Geometry check sheet. Reference: the model listing, model coordinates, mm. A direction names the side the tool comes from. Give positions to 0.01 mm unless a question says otherwise; leave off trailing zeros. Order: outer loops, then holes, each group sorted by start corner. A loop starts at its lowest first (then second) coordinate and runs counter-clockwise, first axis right, second up. Notation, with made-up numbers: M 67,55 L 101,55 A14 ccw 101,69 Z; hole C -19.5,43 d2. An arc over 180 degrees is marked long. Answer as CSV lines item,"result". Start each with the question number.
Q1. Set-up check for faces 1 (the flat face through (2, 4, -1)), 2 (the flat face through (1.8, 3.4, 1.9)), 3 (the flat face through (0, 2, 1)): record each of +Z, -Z, +X, -X, +Y, -Y from which the full face is reachable in a straight line by a thin tool's end or side.
Q2. Go/stop test with flat-tipped pins: pin 1 (1.8 mm diameter, centred on x = 4, z = 2.5, fed in from +Y); pin 2 (0.5 mm diameter, centred on y = 3.5, z = 2.5, fed in from +X); pin 3 (2 mm diameter, centred on x = 4, z = 1.5, fed in from +Y). Record where each tip stops, or that it passes through.
Q3. Thickness scan on line 1 (Y direction, x = 3.7, z = 1); line 2 (Y direction, x = 0.9, z = 1); line 3 (Z direction, x = 4.2, y = 0.25). Record the ranges inside material, lowest first.
Q4. Section check A-A, the plane y = 2.7. Record the boundary of the cut face in (x, z), then the cut area to 3 significant figures.
```python
from build123d import *

# Parameters (mm, degrees)
BOSS_EXTRUDE1_DEPTH = 3.2
BOSS_EXTRUDE2_DEPTH = 1.8
BOSS_EXTRUDE3_DEPTH = 3.2


with BuildPart() as part:
    # Sketch1 → Boss-Extrude1 (new body)
    with BuildSketch(Plane(origin=(0, 0, 0), x_dir=(0, 0, -1), z_dir=(1, 0, 0))):
        with BuildLine():
            Line((2.000388773, 4), (-0.998443773, 4))
            Line((-0.998443773, 4), (-0.998443773, 1.094743417))
            add(Edge.make_bspline(
                [(2.000388773, 0), (0.565989501, 1.139941433), (-0.998443773, 1.094743417)],
                knots=[0, 0, 0, 0.519824709, 0.519824709, 0.519824709], degree=2))
            Line((2.000388773, 0), (2.000388773, 4))
        make_face()
    extrude(amount=BOSS_EXTRUDE1_DEPTH)

    # Sketch2 → Boss-Extrude2 (add)
    with BuildSketch(Plane.ZY):
        with BuildLine():
            add(Edge.make_bspline(
                [(0.998443773, 1.094743417), (2.014440988, 1.074460094), (3.030499337, 0.688991657), (3.999611226, 0)],
                knots=[0.49982829, 0.49982829, 0.49982829, 0.49982829, 1, 1, 1, 1], degree=3))
            Line((3.999611227, 0), (3.999611226, 0.998709843))
            ThreePointArc((3.999611226, 0.998709843), (3.120597073, 3.120899083), (0.998443773, 4))
            Line((0.998443773, 4), (0.998443773, 1.094743417))
        make_face()
    extrude(amount=-BOSS_EXTRUDE2_DEPTH)

    # Sketch3 → Boss-Extrude3 (add)
    with BuildSketch(Plane(origin=(1.8, 0, 0), x_dir=(0, 0, -1), z_dir=(1, 0, 0))):
        with BuildLine():
            add(Edge.make_bspline(
                [(-3.999611227, 0), (-3.02996408, 0.689665176), (-2.014175759, 1.074793835), (-0.998443773, 1.094743417)],
                knots=[0, 0, 0, 0, 0.50017171, 0.50017171, 0.50017171, 0.50017171], degree=3))
            Line((-0.998443773, 1.094743417), (-0.998443773, 3))
            Line((-0.998443773, 3), (-3.234965952, 3))
            ThreePointArc((-3.234965952, 3), (-3.801940417, 2.069905984), (-3.999611226, 0.998709843))
            Line((-3.999611227, 0.998709843), (-3.999611227, 0))
        make_face()
        with BuildLine():
            add(Edge.make_bspline(
                [(-0.998443773, 1.094743417), (0.016590806, 1.114679302), (1.031569126, 0.769937407), (2.000388773, 0)],
                knots=[0.50017171, 0.50017171, 0.50017171, 0.50017171, 1, 1, 1, 1], degree=3))
            Line((2.000388773, 0), (2.000388773, 5.000856569))
            add(Edge.make_bspline(
                [(2.000388773, 5.000856569), (1.39753578, 2.931475432), (-0.998443773, 3)],
                knots=[0, 0, 0, 1, 1, 1], degree=2))
            Line((-0.998443773, 3), (-0.998443773, 1.094743417))
        make_face()
    extrude(amount=BOSS_EXTRUDE3_DEPTH)


solid = part.part
```
Answer block:
1,face 1,"+Z, -X, +Y"
1,face 2,"+Z, +X, +Y"
1,face 3,"+Z, -Z, -X, +Y, -Y"
2,pin 1,"stops at y = 3"
2,pin 2,"stops at x = 1.8"
2,pin 3,"stops at y = 4"
3,line 1,"y = 1.09 to 3"
3,line 2,"y = 1.09 to 4"
3,line 3,"z = -2 to -1.66, 3.62 to 4"
4,outline,"M 0,-2 L 5,-2 L 5,3.47 L 0,3.47 Z"
4,area,"27.4 mm2"
